Geometry check sheet. Reference: the model listing, model coordinates, mm. Face numbers are marked on the shaded views. Round coordinates to 2 decimals unless told otherwise and drop trailing zeros. Order: outer loops, then holes, each group sorted by start corner. A loop starts at its lowest first (then second) coordinate and runs counter-clockwise, first axis right, second up. Notation, with made-up numbers: (-18.75, -18.5) -> (-7.75, -18.5) arc R12 cw to (-7.75, -10.5) -> close; hole circle Ø5 at (-25.75, 17.5). An arc over 180 degrees is marked (long way). Use a Markdown table: item, result. Add a question column.
Item 1: Sectioned sample at A-A, the plane y = 25.4. Record the cut outline in (x, z), and give its area (3 significant figures).
Item 2: Sectioned sample at B-B, the plane z = -3.7. Record the cut outline in (x, y) (3 decimals).
Item 3: Material ranges on probe 1 along X at (y, z) = (25.4, -3.85); probe 2 along Y at (x, z) = (56.5, -1.35); probe 3 along Y at (x, z) = (15, -4.1), recorded low to high. Write a range as [from, to].
Item 4: Gauge pin test, flat ends, axial feed: pin 1 Ø7.5 at (x, y) = (53.975, 25.4) entering from +Z; pin 2 Ø3 at (x, y) = (10, 18.5) entering from +Z; pin 3 Ø5 at (x, y) = (15.875, 25.4) entering from +Z. Record the tip position at first contact, or that the pin passes through.
Item 5: Mould release check, pull along Y, two halves, no side actions. Record for the marked faces 1 and 2: pulls with the +Y half, pulls with the -Y half, needs draft (parallel to the pull), parting line crosses it, or undercut.
Autodesk Inventor part; units mm, degrees
ref_plane "YZ Plane" through (0, 0, 0) normal (1, 0, 0) x (0, 1, 0)
ref_plane "XZ Plane" through (0, 0, 0) normal (0, 1, 0) x (-1, 0, 0)
ref_plane "XY Plane" through (0, 0, 0) normal (0, 0, 1) x (1, 0, 0)
sketch "Sketch1" plane through (0, 0, 0) normal (0, 0, 1) x (1, 0, 0)
  line L0 (0, 0) -> (69.85, 0)
  line L1 (69.85, 0) -> (69.85, 44.45)
  line L2 (69.85, 44.45) -> (0, 44.45)
  line L3 (0, 44.45) -> (0, 0)
  dimension "d0" = 69.85
  dimension "d1" = 44.45
extrude "Extrusion1" add sketch "Sketch1" against normal blind 4.7625
hole "Hole1" at (15.875, 25.4, 0) direction (0, 0, -1) diameter 6.35 end through all countersink diameter 11.4808 countersink angle 82
hole "Hole2" at (53.975, 25.4, 0) direction (0, 0, -1) diameter 6.35 end through all countersink diameter 11.4808 countersink angle 82
properties part number "VS-003 (JAW PLATE)" material "Steel, Alloy"
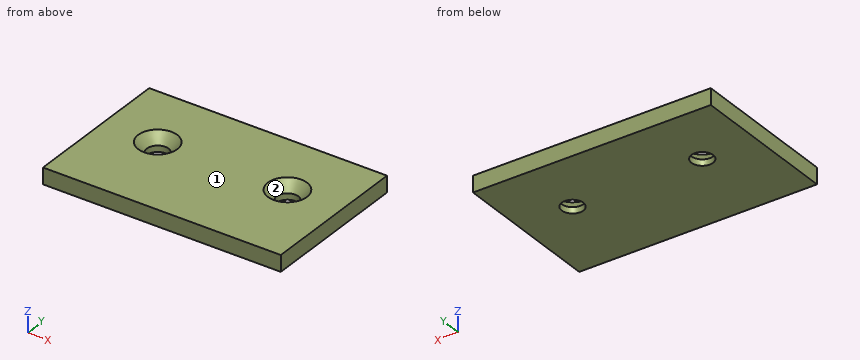
Found:
| question | item | result |
|---|---|---|
| 1 | outline | (0, -4.76) -> (12.7, -4.76) -> (12.7, -2.95) -> (10.13, 0) -> (0, 0) -> close; (19.05, -4.76) -> (50.8, -4.76) -> (50.8, -2.95) -> (48.23, 0) -> (21.62, 0) -> (19.05, -2.95) -> close; (57.15, -4.76) -> (69.85, -4.76) -> (69.85, 0) -> (59.72, 0) -> (57.15, -2.95) -> close |
| 1 | area | 257 mm2 |
| 2 | outline | (0, 0) -> (69.85, 0) -> (69.85, 44.45) -> (0, 44.45) -> close; hole circle Ø6.35 at (15.875, 25.4); hole circle Ø6.35 at (53.975, 25.4) |
| 3 | probe 1 | x = [0, 12.7], [19.05, 50.8], [57.15, 69.85] |
| 3 | probe 2 | y = [0, 21.59], [29.21, 44.45] |
| 3 | probe 3 | y = [0, 22.35], [28.45, 44.45] |
| 4 | pin 1 | stops at z = -2.29 |
| 4 | pin 2 | stops at z = 0 |
| 4 | pin 3 | passes through |
| 5 | face 1 | needs draft |
| 5 | face 2 | undercut |
